```python
from build123d import *

# Parameters (mm, degrees)
SKETCH2_R                                        = 20.32
BOSS_EXTRUDE1_DEPTH                              = 9.525
BOSS_EXTRUDE1_TAPER                              = 1
CUT_EXTRUDE1_DEPTH                               = 1.675
CUT_EXTRUDE2_DEPTH                               = 1.675
CUT_EXTRUDE3_DEPTH                               = 1.675
CUT_EXTRUDE4_DEPTH                               = 1.675
CUT_EXTRUDE5_DEPTH                               = 1.675
CUT_EXTRUDE6_DEPTH                               = 1.675
CUT_EXTRUDE7_DEPTH                               = 1.675
CUT_EXTRUDE8_DEPTH                               = 1.675
SKETCH11_W                                       = 4
SKETCH11_H                                       = 6.374
F_4_4_4_4_DIAMETER_HOLE1_D                       = 4.4
F_4_4_4_4_DIAMETER_HOLE2_D                       = 4.4
CBORE_FOR_M4_HEX_HEAD_MACHINE_SCREW1_D           = 4.3
CBORE_FOR_M4_HEX_HEAD_MACHINE_SCREW1_CBORE_D     = 6.985
CBORE_FOR_M4_HEX_HEAD_MACHINE_SCREW1_CBORE_DEPTH = 1.524
CHAMFER1_SIZE                                    = 0.635014452
CHAMFER1_SIZE2                                   = 0.635014007
CHAMFER2_SIZE                                    = 0.634991023
CHAMFER2_SIZE_2                                  = 0.634990726
CHAMFER3_SIZE                                    = 0.635002922
CHAMFER3_SIZE2                                   = 0.635003014


with BuildPart() as part:
    # Sketch1 → Revolve1 (revolve)
    with BuildSketch(Plane(origin=(0, 0, 0), x_dir=(-1, 0, 0), z_dir=(0, 0, -1)), mode=Mode.PRIVATE) as revolve1_sk:
        Polygon((-30.226, -3.175), (-18.82, -3.175), (-18.764580169, 0), (-30.170580169, 0), align=None)
    revolve(revolve1_sk.sketch.rotate(Axis((0, -3.175, 0), (0, 1, 0)), 270), axis=Axis((0, -3.175, 0), (0, 1, 0)))

    # Sketch2 → Boss-Extrude1 (add)
    with BuildSketch(Plane(origin=(0, 0, 0), x_dir=(-1, 0, 0), z_dir=(0, 1, 0))):
        Circle(SKETCH2_R)
    extrude(amount=BOSS_EXTRUDE1_DEPTH, taper=BOSS_EXTRUDE1_TAPER)

    # Sketch3 → Cut-Extrude1 (cut)
    with BuildSketch(Plane.XZ.offset(3.175)):
        with BuildLine():
            Line((-0.75, 20.30615424), (-0.75, 21.725765386))
            ThreePointArc((-0.75, 21.725765386), (-3.704512163, 24.817685966), (-1.841086622, 28.666940472))
            ThreePointArc((-1.841086622, 28.666940472), (-10.992964278, 26.539363451), (-18.968743169, 21.572432839))
            ThreePointArc((-18.968743169, 21.572432839), (-14.929268369, 20.168239712), (-14.832105945, 15.892766117))
            Line((-14.832105945, 15.892766117), (-13.828289277, 14.888949448))
            ThreePointArc((-13.828289277, 14.888949448), (-7.776127346, 18.773232101), (-0.75, 20.30615424))
        make_face()
    extrude(amount=-CUT_EXTRUDE1_DEPTH, mode=Mode.SUBTRACT)

    # Sketch4 → Cut-Extrude2 (cut)
    with BuildSketch(Plane.XZ.offset(3.175)):
        with BuildLine():
            Line((0.75, 21.725765386), (0.75, 20.30615424))
            ThreePointArc((0.75, 20.30615424), (7.776127346, 18.773232101), (13.828289277, 14.888949448))
            Line((13.828289277, 14.888949448), (14.832105945, 15.892766117))
            ThreePointArc((14.832105945, 15.892766117), (14.929268369, 20.168239712), (18.968743169, 21.572432839))
            ThreePointArc((18.968743169, 21.572432839), (10.992964278, 26.539363451), (1.841086622, 28.666940472))
            ThreePointArc((1.841086622, 28.666940472), (3.704512163, 24.817685966), (0.75, 21.725765386))
        make_face()
    extrude(amount=-CUT_EXTRUDE2_DEPTH, mode=Mode.SUBTRACT)

    # Sketch5 → Cut-Extrude3 (cut)
    with BuildSketch(Plane.XZ.offset(3.175)):
        with BuildLine():
            Line((15.892766117, 14.832105945), (14.888949448, 13.828289277))
            ThreePointArc((14.888949448, 13.828289277), (18.773232101, 7.776127346), (20.30615424, 0.75))
            Line((20.30615424, 0.75), (21.725765386, 0.75))
            ThreePointArc((21.725765386, 0.75), (24.817685966, 3.704512163), (28.666940472, 1.841086622))
            ThreePointArc((28.666940472, 1.841086622), (26.539363451, 10.992964278), (21.572432839, 18.968743169))
            ThreePointArc((21.572432839, 18.968743169), (20.168239712, 14.929268369), (15.892766117, 14.832105945))
        make_face()
    extrude(amount=-CUT_EXTRUDE3_DEPTH, mode=Mode.SUBTRACT)

    # Sketch6 → Cut-Extrude4 (cut)
    with BuildSketch(Plane.XZ.offset(3.175)):
        with BuildLine():
            Line((21.725765386, -0.75), (20.30615424, -0.75))
            ThreePointArc((20.30615424, -0.75), (18.773232101, -7.776127346), (14.888949448, -13.828289277))
            Line((14.888949448, -13.828289277), (15.892766117, -14.832105945))
            ThreePointArc((15.892766117, -14.832105945), (20.168239712, -14.929268369), (21.572432839, -18.968743169))
            ThreePointArc((21.572432839, -18.968743169), (26.539363451, -10.992964278), (28.666940472, -1.841086622))
            ThreePointArc((28.666940472, -1.841086622), (24.817685966, -3.704512163), (21.725765386, -0.75))
        make_face()
    extrude(amount=-CUT_EXTRUDE4_DEPTH, mode=Mode.SUBTRACT)

    # Sketch7 → Cut-Extrude5 (cut)
    with BuildSketch(Plane.XZ.offset(3.175)):
        with BuildLine():
            Line((14.832105945, -15.892766117), (13.828289277, -14.888949448))
            ThreePointArc((13.828289277, -14.888949448), (7.776127346, -18.773232101), (0.75, -20.30615424))
            Line((0.75, -20.30615424), (0.75, -21.725765386))
            ThreePointArc((0.75, -21.725765386), (3.704512163, -24.817685966), (1.841086622, -28.666940472))
            ThreePointArc((1.841086622, -28.666940472), (10.992964278, -26.539363451), (18.968743169, -21.572432839))
            ThreePointArc((18.968743169, -21.572432839), (14.929268369, -20.168239712), (14.832105945, -15.892766117))
        make_face()
    extrude(amount=-CUT_EXTRUDE5_DEPTH, mode=Mode.SUBTRACT)

    # Sketch8 → Cut-Extrude6 (cut)
    with BuildSketch(Plane.XZ.offset(3.175)):
        with BuildLine():
            Line((-0.75, -21.725765386), (-0.75, -20.30615424))
            ThreePointArc((-0.75, -20.30615424), (-7.776127346, -18.773232101), (-13.828289277, -14.888949448))
            Line((-13.828289277, -14.888949448), (-14.832105945, -15.892766117))
            ThreePointArc((-14.832105945, -15.892766117), (-14.929268369, -20.168239712), (-18.968743169, -21.572432839))
            ThreePointArc((-18.968743169, -21.572432839), (-10.992964278, -26.539363451), (-1.841086622, -28.666940472))
            ThreePointArc((-1.841086622, -28.666940472), (-3.704512163, -24.817685966), (-0.75, -21.725765386))
        make_face()
    extrude(amount=-CUT_EXTRUDE6_DEPTH, mode=Mode.SUBTRACT)

    # Sketch9 → Cut-Extrude7 (cut)
    with BuildSketch(Plane.XZ.offset(3.175)):
        with BuildLine():
            Line((-15.892766117, -14.832105945), (-14.888949448, -13.828289277))
            ThreePointArc((-14.888949448, -13.828289277), (-18.773232101, -7.776127346), (-20.30615424, -0.75))
            Line((-20.30615424, -0.75), (-21.725765386, -0.75))
            ThreePointArc((-21.725765386, -0.75), (-24.817685966, -3.704512163), (-28.666940472, -1.841086622))
            ThreePointArc((-28.666940472, -1.841086622), (-26.539363451, -10.992964278), (-21.572432839, -18.968743169))
            ThreePointArc((-21.572432839, -18.968743169), (-20.168239712, -14.929268369), (-15.892766117, -14.832105945))
        make_face()
    extrude(amount=-CUT_EXTRUDE7_DEPTH, mode=Mode.SUBTRACT)

    # Sketch10 → Cut-Extrude8 (cut)
    with BuildSketch(Plane.XZ.offset(3.175)):
        with BuildLine():
            Line((-21.725765386, 0.75), (-20.30615424, 0.75))
            ThreePointArc((-20.30615424, 0.75), (-18.773232101, 7.776127346), (-14.888949448, 13.828289277))
            Line((-14.888949448, 13.828289277), (-15.892766117, 14.832105945))
            ThreePointArc((-15.892766117, 14.832105945), (-20.168239712, 14.929268369), (-21.572432839, 18.968743169))
            ThreePointArc((-21.572432839, 18.968743169), (-26.539363451, 10.992964278), (-28.666940472, 1.841086622))
            ThreePointArc((-28.666940472, 1.841086622), (-24.817685966, 3.704512163), (-21.725765386, 0.75))
        make_face()
    extrude(amount=-CUT_EXTRUDE8_DEPTH, mode=Mode.SUBTRACT)

    # Sketch11 → Revolve2 (revolve)
    with BuildSketch(Plane.XY, mode=Mode.PRIVATE) as revolve2_sk:
        with Locations((2, 4.838)):
            Rectangle(SKETCH11_W, SKETCH11_H)
    revolve(revolve2_sk.sketch.rotate(Axis((0, 8.025, 0), (0, -1, 0)), 90), axis=Axis((0, 8.025, 0), (0, -1, 0)))

    # Ø4.4 (4.4) Diameter Hole1 (through all)
    with Locations(Plane(origin=(0, 0, 0), x_dir=(1, 0, 0), z_dir=(0, 1, 0))):
        with Locations((25.4, 0), (17.960512242, 17.960512242), (0, 25.4), (-17.960512242, 17.960512242), (-25.4, 0), (-17.960512242, -17.960512242), (0, -25.4), (17.960512242, -17.960512242)):
            Hole(F_4_4_4_4_DIAMETER_HOLE1_D / 2)

    # Ø4.4 (4.4) Diameter Hole2 (through all)
    with Locations(Plane(origin=(0, 9.525, 0), x_dir=(1, 0, 0), z_dir=(0, 1, 0))):
        with Locations((12.7, 0), (0, 12.7), (-12.7, 0), (0, -12.7)):
            Hole(F_4_4_4_4_DIAMETER_HOLE2_D / 2)

    # CBORE for M4 Hex Head Machine Screw1 (through all)
    with Locations(Plane(origin=(0, 9.525, 0), x_dir=(1, 0, 0), z_dir=(0, 1, 0))):
        with Locations((0, 0)):
            CounterBoreHole(CBORE_FOR_M4_HEX_HEAD_MACHINE_SCREW1_D / 2, CBORE_FOR_M4_HEX_HEAD_MACHINE_SCREW1_CBORE_D / 2, CBORE_FOR_M4_HEX_HEAD_MACHINE_SCREW1_CBORE_DEPTH)

    # Chamfer1
    chamfer1_edges = [part.edges().sort_by_distance(p)[0] for p in [
        (20.32, 0, 0),
    ]]
    chamfer1_side = [part.faces().sort_by_distance(p)[0] for p in [
        (0, 0, -29.317227296),
    ]]
    chamfer(chamfer1_edges, length=CHAMFER1_SIZE, length2=CHAMFER1_SIZE2, reference=chamfer1_side[0])

    # Chamfer2
    # the kernel refuses this chamfer: 0.634991023, 0.634990726 mm, written as the material it takes off along each edge
    with BuildSketch(Plane(origin=(0, 9.525, 0), x_dir=(-1, 0, 0), z_dir=(0, 0, 1))) as chamfer2_piece_1:
        Polygon((20.153740507 + CHAMFER2_SIZE * 0.0174524064387, CHAMFER2_SIZE * 0.999847695238), (20.153740507 - CHAMFER2_SIZE_2, 0), (20.153740507, 0), align=None)
    revolve(axis=Axis((0, 9.525, 0), (0, -1, 0)), mode=Mode.SUBTRACT)

    # Chamfer3
    chamfer3_edges = [part.edges().sort_by_distance(p)[0] for p in [
        (0, 0, -30.170580169),
    ]]
    chamfer3_side = [part.faces().sort_by_distance(p)[0] for p in [
        (21.808367326, 0, 0),
    ]]
    chamfer(chamfer3_edges, length=CHAMFER3_SIZE, length2=CHAMFER3_SIZE2, reference=chamfer3_side[0])


solid = part.part
```
The listing builds one solid part. Answer for the finished solid, in the listing's coordinates (mm). A direction names the side the tool comes from. Round coordinates to 2 decimals unless told otherwise and drop trailing zeros. Loops run counter-clockwise (first coordinate to the right, second up) from the corner with the lowest first, then second, coordinate; pieces in that order, holes last. Notation, with made-up numbers: (4.5, 58.5) - (23.5, 58.5) arc R14 ccw to (23.5, 84.5) - close; hole circle Ø3 at (-13.75, 75). An arc over 180 degrees is marked (long way). Return JSON: item names as keys, results as strings. Group by question number.
1. The part is cut by section A-A on y = 1.75. Determine the outline of the cut face in (x, z).
2. The mould has two halves that part along Z. Classify faces 1 (the cylindrical face through (-11.11, -2.35, -26.49)), 2 (the flat face through (20, 0, 9)), 3 (the conical face through (20.41, -1.36, -22.25)), 4 (the cylindrical face through (24.881, -2.349, -3.714)): pulls with the +Z half, pulls with the -Z half, needs draft (parallel to the pull), parting line crosses it, or undercut.
3. The part is cut by section C-C on y = 6. Determine the outline of the cut face in (x, z), then the cut area to 3 significant figures.
4. The part is cut by section B-B on z = 0. State how many separate pieces and enclosed holes the cut face has, then the cut area to 3 significant figures.
5. Which of the six approach directions +Z, -Z, +X, -X, +Y, -Y give full straight-line access (tool end or side, diameter ignored) to faces 5 (the cylindrical face through (-19.993, -1.61, 18.803)), 6 (the cylindrical face through (-7.683, -2.349, -18.812))?
6. Consider probe 1 along Z at (x, y) = (3, -2); probe 2 along Y at (x, z) = (-7.5, 0.5) (3 decimals); probe 3 along Y at (x, z) = (-26.5, 6.5). Determine where each line is inside the solid, lowest interval first.
7. Each of these flat-tipped pins is pushed along its axis until it touches: P1, Ø3.5, axis at x = 25.4, z = 0, coming from the -Y side; P2, Ø2, axis at x = 12, y = 0, coming from the -Z side; P3, Ø4, axis at x = -15.5, z = -3, coming from the -Y side; P4, Ø2, axis at x = 22, z = -17.5, coming from the +Y side. Where does it stop, or does it pass through?
Resolved:
{
 "1": {"outline": "circle Ø40.58 at (0, 0); hole circle Ø4.4 at (-12.7, 0); hole circle Ø4.4 at (0, -12.7); hole circle Ø4.4 at (0, 12.7); hole circle Ø4.3 at (0, 0); hole circle Ø4.4 at (12.7, 0)"},
 "2": {"face 1": "undercut", "face 2": "needs draft", "face 3": "parting line crosses it", "face 4": "undercut"},
 "3": {"outline": "circle Ø40.43 at (0, 0); hole circle Ø4.4 at (-12.7, 0); hole circle Ø4.4 at (0, -12.7); hole circle Ø4.4 at (0, 12.7); hole circle Ø4.3 at (0, 0); hole circle Ø4.4 at (12.7, 0)", "area": "1,210 mm²"},
 "4": {"separate pieces": "6", "enclosed holes": "0", "area": "301 mm²"},
 "5": {"face 5": "+Y, -Y", "face 6": "-Y"},
 "6": {"probe 1": "z = -30.06 to -28.57, -27.65 to -23.15, -20.1 to -18.56, 18.56 to 20.1, 23.15 to 27.65, 28.57 to 30.06", "probe 2": "y = 0 to 9.525", "probe 3": "y = -1.5 to 0"},
 "7": {"P1": "passes through", "P2": "stops at z = -28.02", "P3": "stops at y = 0", "P4": "stops at y = 0"}
}
